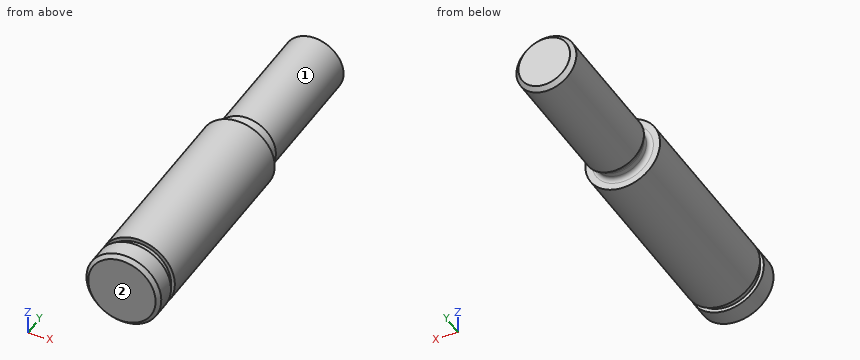
```python
from build123d import *

# Parameters (mm, degrees)
SKETCH1_R           = 5
BOSS_EXTRUDE1_DEPTH = 50
CHAMFER1_SIZE       = 0.5
CUT_EXTRUDE2_START  = -3
SKETCH7_R           = 5
SKETCH7_R_2         = 4.5
CUT_EXTRUDE2_DEPTH  = 1


# Read off the part's stored shape, not the designer's step: M8x1.0 Machine Threads Stud1
with BuildPart() as part:
    # Sketch1 → Boss-Extrude1 (new body)
    with BuildSketch(Plane(origin=(0, 0, 0), x_dir=(1, 0, 0), z_dir=(0, 1, 0))):
        with Locations(Location((0, 0, 0), (0, 0, 270))):
            Circle(SKETCH1_R)
    extrude(amount=BOSS_EXTRUDE1_DEPTH)

    # M8x1.0 Machine Threads Stud1 outline → M8x1.0 Machine Threads Stud1 (revolve, cut)
    with BuildSketch(Plane.XY):
        with BuildLine():
            Line((5, 50), (3.4455, 50))
            Line((3.4455, 50), (4, 49.4455))
            Line((4, 49.4455), (4, 32))
            Line((4, 32), (3.580384758, 31.273205081))
            ThreePointArc((3.580384758, 31.273205081), (3.520444504, 31.128496508), (3.5, 30.973205081))
            Line((3.5, 30.973205081), (3.5, 30.373205081))
            ThreePointArc((3.5, 30.373205081), (3.675735931, 29.948941012), (4.1, 29.773205081))
            Line((4.1, 29.773205081), (5, 29.773205081))
            Line((5, 29.773205081), (5, 50))
        make_face()
    revolve(axis=Axis((0, 0, 0), (0, 1, 0)), mode=Mode.SUBTRACT)

    # Chamfer1
    chamfer1_edges = [part.edges().sort_by_distance(p)[0] for p in [
        (0, 0, -5),
    ]]
    chamfer(chamfer1_edges, length=CHAMFER1_SIZE)

    # Sketch7 → Cut-Extrude2 (cut)
    with BuildSketch(Plane.XZ.offset(CUT_EXTRUDE2_START)):
        with Locations(Location((0, 0, 0), (0, 0, 270))):
            Circle(SKETCH7_R)
        with Locations(Location((0, 0, 0), (0, 0, 270))):
            Circle(SKETCH7_R_2, mode=Mode.SUBTRACT)
    extrude(amount=-CUT_EXTRUDE2_DEPTH, mode=Mode.SUBTRACT)


solid = part.part
```
Could you check a few things on this model? Use its own coordinates, in mm. Face numbers are marked on the shaded views. A direction names the side the tool comes from. Round coordinates to 2 decimals unless told otherwise and drop trailing zeros. Write each loop counter-clockwise with the first axis right and the second up, starting at its lowest first coordinate (ties: lowest second). Pieces come first, ordered by that corner, then holes.
(1) If I drill on probe 1 along Y at (x, z) = (-2, 4); probe 2 along Z at (x, y) = (-0.25, 48); probe 3 along X at (y, z) = (35, 0), over which ranges is the centre line in solid material (lowest first)?
Findings below:
probe 1: y = 0 to 29.77
probe 2: z = -3.99 to 3.99
probe 3: x = -4 to 4
(2) Suppose I cut it at B-B on x = 0. Write out the boundary of the cut face in (y, z).
Findings below:
outline: (0, -4.5) - (0.5, -5) - (3, -5) - (3, -4.5) - (4, -4.5) - (4, -5) - (29.77, -5) - (29.77, -4.1) arc R0.6 cw to (30.37, -3.5) - (30.97, -3.5) arc R0.6 cw to (31.27, -3.58) - (32, -4) - (49.45, -4) - (50, -3.45) - (50, 3.45) - (49.45, 4) - (32, 4) - (31.27, 3.58) arc R0.6 cw to (30.97, 3.5) - (30.37, 3.5) arc R0.6 cw to (29.77, 4.1) - (29.77, 5) - (4, 5) - (4, 4.5) - (3, 4.5) - (3, 5) - (0.5, 5) - (0, 4.5) - close
(3) Which directions (+Z, -Z, +X, -X, +Y, -Y) give clear straight access to the entire face, cutting with the end or side of a thin tool? Please do the marked faces 1 and 2.
Findings below:
face 1: +Y
face 2: +Z, -Z, +X, -X, -Y
(4) For pin 1 (1.5 mm diameter, centred on y = 16, z = -2.5, fed in from -X); pin 2 (2 mm diameter, centred on x = 2, z = 2, fed in from -Y); pin 3 (1.5 mm diameter, centred on y = 17, z = 3.5, fed in from +X); pin 4 (3 mm diameter, centred on x = 2.5, y = 23, fed in from +Z), each with a flat end and sliding along its axis, tell me the tip position at first contact or that it passes through.
Findings below:
pin 1: stops at x = -4.68
pin 2: stops at y = 0
pin 3: stops at x = 4.18
pin 4: stops at z = 4.9
(5) Suppose I cut it at A-A on z = 0. Write out the boundary of the cut face in (x, y), and give its area (3 significant figures).
Findings below:
outline: (-5, 0.5) - (-4.5, 0) - (4.5, 0) - (5, 0.5) - (5, 3) - (4.5, 3) - (4.5, 4) - (5, 4) - (5, 29.77) - (4.1, 29.77) arc R0.6 cw to (3.5, 30.37) - (3.5, 30.97) arc R0.6 cw to (3.58, 31.27) - (4, 32) - (4, 49.45) - (3.45, 50) - (-3.45, 50) - (-4, 49.45) - (-4, 32) - (-3.58, 31.27) arc R0.6 cw to (-3.5, 30.97) - (-3.5, 30.37) arc R0.6 cw to (-4.1, 29.77) - (-5, 29.77) - (-5, 4) - (-4.5, 4) - (-4.5, 3) - (-5, 3) - close
area: 456 mm2
(6) Suppose I cut it at C-C on y = 36. Write out the boundary of the cut face in (x, z).
Findings below:
outline: circle Ø8 at (0, 0)
